Work out the finished part from the listing and answer in its coordinate system (mm). A direction names the side the tool comes from. Give positions to 0.01 mm unless a question says otherwise; leave off trailing zeros. Loops run counter-clockwise (first coordinate to the right, second up) from the corner with the lowest first, then second, coordinate; pieces in that order, holes last. Notation, with made-up numbers: (76.25, -5) - (98.25, -5) arc R6 ccw to (98.25, 1) - close; hole circle Ø3 at (33.25, 77). An arc over 180 degrees is marked (long way). One line per item, written item: value.
from build123d import *

# Parameters (mm, degrees)
SKICA1_W                 = 46
SKICA1_H                 = 24
SKICA1_R                 = 4
P_IDAT_VYSUNUT_M1_DEPTH  = 4
SKICA2_W                 = 30
SKICA2_H                 = 5
ODEBRAT_VYSUNUT_M1_DEPTH = 1


with BuildPart() as part:
    # Skica1 → Přidat vysunutím1 (new body)
    with BuildSketch(Plane.XY):
        Rectangle(SKICA1_W, SKICA1_H)
        with Locations((-15, -5)):
            Circle(SKICA1_R, mode=Mode.SUBTRACT)
        with Locations((-5, -5)):
            Circle(SKICA1_R, mode=Mode.SUBTRACT)
        with Locations((5, -5)):
            Circle(SKICA1_R, mode=Mode.SUBTRACT)
        with Locations((15, -5)):
            Circle(SKICA1_R, mode=Mode.SUBTRACT)
        with Locations((-5, 5)):
            Circle(SKICA1_R, mode=Mode.SUBTRACT)
        with Locations((5, 5)):
            Circle(SKICA1_R, mode=Mode.SUBTRACT)
        with Locations((15, 5)):
            Circle(SKICA1_R, mode=Mode.SUBTRACT)
        with Locations((-15, 5)):
            Circle(SKICA1_R, mode=Mode.SUBTRACT)
    extrude(amount=P_IDAT_VYSUNUT_M1_DEPTH)

    # Skica2 → Odebrat vysunutím1 (cut)
    with BuildSketch(Plane.XY.offset(4)):
        with Locations((0, 5)):
            Rectangle(SKICA2_W, SKICA2_H)
        with Locations((0, -5)):
            Rectangle(SKICA2_W, SKICA2_H)
    extrude(amount=-ODEBRAT_VYSUNUT_M1_DEPTH, mode=Mode.SUBTRACT)


solid = part.part
1. Section B-B (y = 5) is taken. Write down the section's boundary in (x, z).
Output:
outline: (-23, 0) - (-19, 0) - (-19, 4) - (-23, 4) - close; (-11, 0) - (-9, 0) - (-9, 3) - (-11, 3) - close; (-1, 0) - (1, 0) - (1, 3) - (-1, 3) - close; (9, 0) - (11, 0) - (11, 3) - (9, 3) - close; (19, 0) - (23, 0) - (23, 4) - (19, 4) - close
2. For faces 4 (the cylindrical face through (-19, -5, 2)), 5 (the flat face through (10, -7.5, 3.5)), determine the directions among +Z, -Z, +X, -X, +Y, -Y from which every point of the face is accessible in a straight line to the end or side of a thin tool.
Output:
face 4: +Z, -Z
face 5: +Z
3. Flat-ended cylindrical pins translate along their axes: pin 1 Ø12 at (x, y) = (-10.5, 8.5) entering from -Z; pin 2 Ø6.5 at (x, y) = (-15, 5) entering from +Z; pin 3 Ø1.9 at (x, y) = (1, -4) entering from +Z. Find the tip coordinate at first contact, or state that the pin passes through.
Output:
pin 1: stops at z = 0
pin 2: passes through
pin 3: stops at z = 3
4. Find the intervals of material crossed by line 1 along Y through (x, z) = (-5, 2); line 2 along X through (y, z) = (5, 2.4); line 3 along Y through (x, z) = (-12.5, 0.5), in increasing order.
Output:
line 1: y = -12 to -9, -1 to 1, 9 to 12
line 2: x = -23 to -19, -11 to -9, -1 to 1, 9 to 11, 19 to 23
line 3: y = -12 to -8.12, -1.88 to 1.88, 8.12 to 12
5. Section D-D (x = 6.5) is taken. Write down the section's boundary in (y, z), and give its area (3 significant figures).
Output:
outline: (-12, 0) - (-8.71, 0) - (-8.71, 4) - (-12, 4) - close; (-1.29, 0) - (1.29, 0) - (1.29, 4) - (-1.29, 4) - close; (8.71, 0) - (12, 0) - (12, 4) - (8.71, 4) - close
area: 36.7 mm²
6. The mould has two halves that part along Y. Classify faces 1 (the cylindrical face through (-19, 5, 2)), 2 (the flat face through (-23, 0, 2)), 3 (the flat face through (0, 12, 2)): released by +Y, released by -Y, zero draft, split by the parting line, or undercut.
Output:
face 1: undercut
face 2: zero draft
face 3: released by +Y
7. Section A-A (x = -5) is taken. Write down the section's boundary in (y, z).
Output:
outline: (-12, 0) - (-9, 0) - (-9, 4) - (-12, 4) - close; (-1, 0) - (1, 0) - (1, 4) - (-1, 4) - close; (9, 0) - (12, 0) - (12, 4) - (9, 4) - close
8. Section C-C (z = 1.2) is taken. Count the separate pieces of the cut face and the enclosed holes in it, and give its area (3 significant figures).
Output:
separate pieces: 1
enclosed holes: 8
area: 702 mm²
